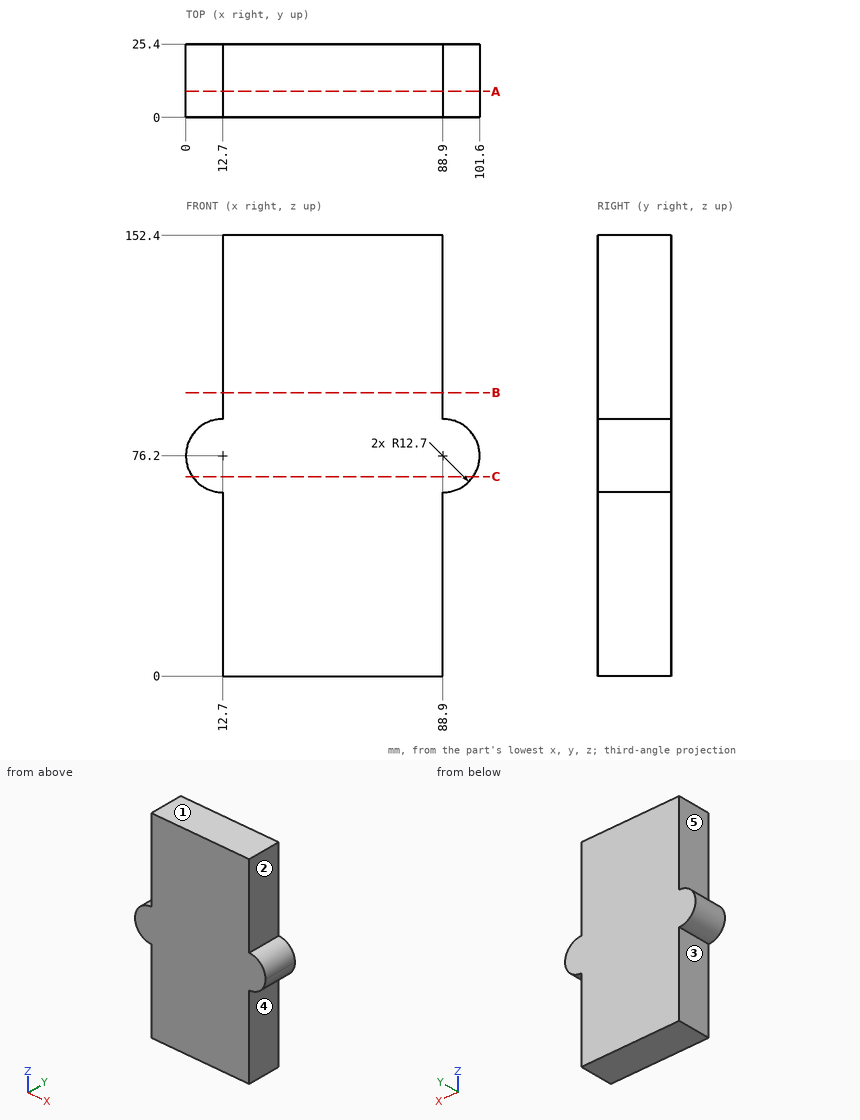
The drawing under review shows one solid part. Ordinate dimensions are in mm from its lowest x, y, z. A direction names the side the tool comes from. Round coordinates to 2 decimals unless told otherwise and drop trailing zeros. Write each loop counter-clockwise with the first axis right and the second up, starting at its lowest first coordinate (ties: lowest second). Pieces come first, ordered by that corner, then holes. Notation, with made-up numbers: (-21, 50) - (23, 50) arc R12 ccw to (23, 57) - close; hole circle Ø10 at (61.25, 85.25). An arc over 180 degrees is marked (long way). Use a Markdown table: item, result. Add a question column.
1. We need section A-A (y = 9). State the section outline as (x, z) points.
2. Clearance check with flat-ended pins moving along their axes: pin 1 (7.5 mm diameter, centred on y = 17.5, z = 26, fed in from +X); pin 2 (1.5 mm diameter, centred on y = 18, z = 85.5, fed in from -X); pin 3 (12.5 mm diameter, centred on y = 7, z = 18, fed in from -X). State where each tip first meets the part, or that it passes through.
3. We need section C-C (z = 69). State the section outline as (x, y) points.
4. For the marked faces 1, 2, 3, 4 and 5, list the 3-axis set-ups (+Z, -Z, +X, -X, +Y, -Y) from which the entire face can be reached by the end or side of a thin tool; tool diameter is ignored.
5. Wall thickness on probe 1 along X at (y, z) = (10.25, 50.5); probe 2 along Z at (x, y) = (91.5, 14): over which ranges is each line inside the solid? List them lowest first.
6. We need section B-B (z = 98). State the section outline as (x, y) points.
Output:
| question | item | result |
|---|---|---|
| 1 | outline | (12.7, 0) - (88.9, 0) - (88.9, 63.5) arc R12.7 ccw to (88.9, 88.9) - (88.9, 152.4) - (12.7, 152.4) - (12.7, 88.9) arc R12.7 ccw to (12.7, 63.5) - close |
| 2 | pin 1 | stops at x = 88.9 |
| 2 | pin 2 | stops at x = 3.31 |
| 2 | pin 3 | stops at x = 12.7 |
| 3 | outline | (2.24, 0) - (99.36, 0) - (99.36, 25.4) - (2.24, 25.4) - close |
| 4 | face 1 | +Z, +X, -X, +Y, -Y |
| 4 | face 2 | +Z, +X, +Y, -Y |
| 4 | face 3 | -Z, -X, +Y, -Y |
| 4 | face 4 | -Z, +X, +Y, -Y |
| 4 | face 5 | +Z, -X, +Y, -Y |
| 5 | probe 1 | x = 12.7 to 88.9 |
| 5 | probe 2 | z = 63.77 to 88.63 |
| 6 | outline | (12.7, 0) - (88.9, 0) - (88.9, 25.4) - (12.7, 25.4) - close |
